Source: CAD feature listing. Evaluate the final solid. Frame: model axes, mm. A direction names the side the tool comes from. Round coordinates to 2 decimals unless told otherwise and drop trailing zeros. Write each loop counter-clockwise with the first axis right and the second up, starting at its lowest first coordinate (ties: lowest second). Pieces come first, ordered by that corner, then holes.
from build123d import *

# Parameters (mm, degrees)
SKETCH1_R           = 20
BOSS_EXTRUDE1_DEPTH = 20
SKETCH2_R           = 2.5
CUT_EXTRUDE1_DEPTH  = 12
FILLET1_R           = 0.79375
SKETCH3_R           = 17
SKETCH3_R_2         = 9
CUT_EXTRUDE2_DEPTH  = 0.79375


with BuildPart() as part:
    # Sketch1 → Boss-Extrude1 (new body)
    with BuildSketch(Plane(origin=(0, 0, 0), x_dir=(1, 0, 0), z_dir=(0, 1, 0))):
        Circle(SKETCH1_R)
    extrude(amount=BOSS_EXTRUDE1_DEPTH)

    # Sketch2 → Cut-Extrude1 (cut)
    with BuildSketch(Plane(origin=(0, 20, 0), x_dir=(1, 0, 0), z_dir=(0, 1, 0))):
        Circle(SKETCH2_R)
    extrude(amount=-CUT_EXTRUDE1_DEPTH, mode=Mode.SUBTRACT)

    # Fillet1
    fillet1_edges = [part.edges().sort_by_distance(p)[0] for p in [
        (-20, 0, 0),
        (-20, 20, 0),
    ]]
    fillet(fillet1_edges, radius=FILLET1_R)

    # Sketch3 → Cut-Extrude2 (cut)
    with BuildSketch(Plane.XZ):
        Circle(SKETCH3_R)
        Circle(SKETCH3_R_2, mode=Mode.SUBTRACT)
    extrude(amount=-CUT_EXTRUDE2_DEPTH, mode=Mode.SUBTRACT)


solid = part.part
1) Contact query for flat-ended pins moving along their axis: P1, Ø8, axis at y = 16, z = 12, coming from the +X side; P2, Ø5, axis at y = 6, z = 15.5, coming from the +X side; P3, Ø2, axis at x = 13.5, y = 11.5, coming from the -Z side. Output: stop coordinate, or through.
Taken from the geometry:
P1: stops at x = 18.33
P2: stops at x = 15.2
P3: stops at z = -15.61
2) Material intervals for line 1 (X direction, y = 14.75, z = 0); line 2 (Z direction, x = 0, y = 0.35), sorted ascending.
Taken from the geometry:
line 1: x = -20 to -2.5, 2.5 to 20
line 2: z = -19.86 to -17, -9 to 9, 17 to 19.86
3) Section query C-C on y = 9. Return the cut outline in (x, z).
Taken from the geometry:
outline: circle Ø40 at (0, 0); hole circle Ø5 at (0, 0)
4) Pull-direction query (X, two-part tool) for faces 1 (the face through (0, 20, 4)), 2 (the face through (-4.336, 9.871, 19.524)), 3 (the face through (0, 8, 0)); classes: released by +X, released by -X, zero draft, split by the parting line, or undercut.
Taken from the geometry:
face 1: zero draft
face 2: split by the parting line
face 3: undercut
5) Section query D-D on y = 6.5. Return the cut outline in (x, z), then the cut area to 3 significant figures.
Taken from the geometry:
outline: circle Ø40 at (0, 0)
area: 1,260 mm2
6) Section query B-B on z = 0. Return the cut outline in (x, y), then the cut area to 3 significant figures.
Taken from the geometry:
outline: (-20, 0.79) arc R0.79 ccw to (-19.21, 0) - (-17, 0) - (-17, 0.79) - (-9, 0.79) - (-9, 0) - (9, 0) - (9, 0.79) - (17, 0.79) - (17, 0) - (19.21, 0) arc R0.79 ccw to (20, 0.79) - (20, 19.21) arc R0.79 ccw to (19.21, 20) - (2.5, 20) - (2.5, 8) - (-2.5, 8) - (-2.5, 20) - (-19.21, 20) arc R0.79 ccw to (-20, 19.21) - close
area: 727 mm2
7) Section query A-A on x = 0. Return the cut outline in (y, z), then the cut area to 3 significant figures.
Taken from the geometry:
outline: (0, -19.21) arc R0.79 ccw to (0.79, -20) - (19.21, -20) arc R0.79 ccw to (20, -19.21) - (20, -2.5) - (8, -2.5) - (8, 2.5) - (20, 2.5) - (20, 19.21) arc R0.79 ccw to (19.21, 20) - (0.79, 20) arc R0.79 ccw to (0, 19.21) - (0, 17) - (0.79, 17) - (0.79, 9) - (0, 9) - (0, -9) - (0.79, -9) - (0.79, -17) - (0, -17) - close
area: 727 mm2
8) Reachability of faces 4 (the face through (-0.54, 14.08, 2.44)), 5 (the face through (-1.172, 0.391, 8.923)), 6 (the face through (0, 0, 0)) from +Z, -Z, +X, -X, +Y, -Y: full face, straight path, thin tool, end or side. Return the list, or none.
Taken from the geometry:
face 4: +Y
face 5: -Y
face 6: +Z, -Z, +X, -X, -Y
